```python
from build123d import *

# Parameters (mm, degrees)
F2_DEPTH = 5


with BuildPart() as f2:
    # F1 (on Right) → F2 (new body)
    with BuildSketch(Plane.YZ):
        Polygon((0, 5), (0, 0), (31.5, 0), (31.5, -5), (36.5, -5), (36.5, 0), (45, 0), (45, 2), (43.75, 2), (43.75, 5), (45, 5), (45, 6), (48, 6), (48, 5), (49.25, 5), (49.25, 2), (48, 2), (48, 0), (56.5, 0), (56.5, -5), (61.5, -5), (61.5000001655, 0), (93, 0), (93, 5), (98, 5), (98, 10), (93, 10), (93, 18.5), (91, 18.5), (91, 17.25), (88, 17.25), (88, 18.5), (87, 18.5), (87, 21.5), (88, 21.5), (88, 22.75), (91, 22.75), (91, 21.5), (93, 21.5), (93, 30), (98, 30), (98, 35), (93, 35), (93, 40), (93, 50), (0, 50), (0, 40), (0, 35), (-5, 35), (-5, 30), (0, 30), (0, 21.5), (2, 21.5), (2, 22.75), (5, 22.75), (5, 21.5), (6, 21.5), (6, 18.5), (5, 18.5), (5, 17.25), (2, 17.25), (2, 18.5), (0, 18.5), (0, 10), (-5, 10), (-5, 5), align=None)
        Polygon((36.5, 45), (56.5, 45), (56.5, 40), (45, 40), (36.5, 40), align=None, mode=Mode.SUBTRACT)
    extrude(amount=F2_DEPTH)


solid = f2.part
```
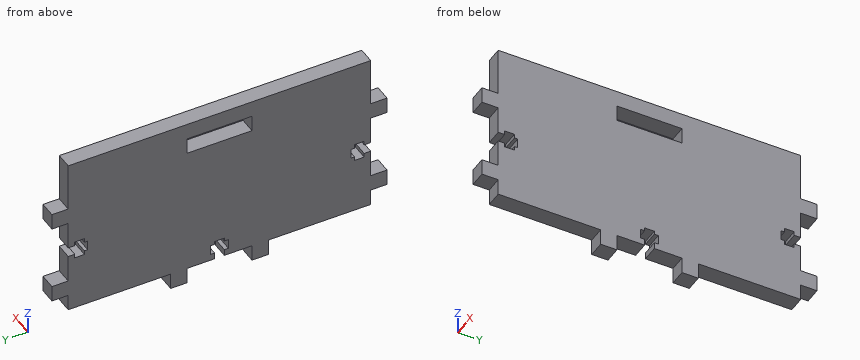
Build history of the part. All positions in model axes, mm. Round coordinates to 2 decimals unless told otherwise and drop trailing zeros. Order: outer loops, then holes, each group sorted by start corner. A loop starts at its lowest first (then second) coordinate and runs counter-clockwise, first axis right, second up. Notation, with made-up numbers: (69.5, 17.25) -> (83.5, 17.25) arc R25 cw to (83.5, 36.25) -> close; hole circle Ø4 at (-6.75, -14). An arc over 180 degrees is marked (long way). Answer in a Markdown table with one row per item.
1) Band-saw the part on C-C on y = 12.5. Give the cut face in (x, z).
Values:
| item | result |
|---|---|
| outline | (0, 0) -> (5, 0) -> (5, 50) -> (0, 50) -> close |
2) Band-saw the part on B-B on z = 41. Give the cut face in (x, y), and give its area (3 significant figures).
Values:
| item | result |
|---|---|
| outline | (0, 0) -> (5, 0) -> (5, 36.5) -> (0, 36.5) -> close; (0, 56.5) -> (5, 56.5) -> (5, 93) -> (0, 93) -> close |
| area | 365 mm2 |
3) Wall check: L1, parallel to Z at x = 3.25, y = 53; L2, parallel to Z at x = 2.1, y = 0.5; L3, parallel to Y at x = 3.4, z = 42.5. Give the ranges that are in metal, low to high.
Values:
| item | result |
|---|---|
| L1 | 0 to 40, 45 to 50 |
| L2 | 0 to 18.5, 21.5 to 50 |
| L3 | 0 to 36.5, 56.5 to 93 |
4) Pin check, flat tips, straight feed: P1, Ø1.5, axis at x = 2.5, y = 40.5, coming from the -Z side; P2, Ø0.9, axis at x = 3.5, z = 20.5, coming from the -Y side; P3, Ø2.5, axis at x = 2, z = 3.5, coming from the +Y side. Stop position of each tip, or through.
Values:
| item | result |
|---|---|
| P1 | z = 0 |
| P2 | y = 6 |
| P3 | y = 93 |
5) Band-saw the part on A-A on y = 46. Give the cut face in (x, z), and give its area (3 significant figures).
Values:
| item | result |
|---|---|
| outline | (0, 6) -> (5, 6) -> (5, 40) -> (0, 40) -> close; (0, 45) -> (5, 45) -> (5, 50) -> (0, 50) -> close |
| area | 195 mm2 |
